Geometry: final body of the model. Coordinates: model frame, mm. A direction names the side the tool comes from. Give positions to 0.01 mm unless a question says otherwise; leave off trailing zeros. Write each loop counter-clockwise with the first axis right and the second up, starting at its lowest first coordinate (ties: lowest second). Pieces come first, ordered by that corner, then holes. Notation, with made-up numbers: M 71,86 L 89,86 A26 ccw 89,123 Z; hole C -36,56 d1. An arc over 180 degrees is marked long. Answer as a JSON object with one key per item and string values.
from build123d import *

# Parameters (mm, degrees)
BASE_EXTRUDE_DEPTH  = 60
CUT_EXTRUDE1_DEPTH  = 50
SKETCH3_R           = 9
BOSS_EXTRUDE1_DEPTH = 15


with BuildPart() as part:
    # Sketch1 → Base-Extrude (new body)
    with BuildSketch(Plane.XY):
        with BuildLine():
            Line((15, 0), (135, 0))
            ThreePointArc((135, 0), (145.606601718, 4.393398282), (150, 15))
            Line((150, 15), (150, 85))
            ThreePointArc((150, 85), (145.606601718, 95.606601718), (135, 100))
            Line((135, 100), (15, 100))
            ThreePointArc((15, 100), (4.393398282, 95.606601718), (0, 85))
            Line((0, 85), (0, 15))
            ThreePointArc((0, 15), (4.393398282, 4.393398282), (15, 0))
        make_face()
    extrude(amount=BASE_EXTRUDE_DEPTH)

    # Sketch2 → Cut-Extrude1 (cut)
    with BuildSketch(Plane.XY.offset(60)):
        with BuildLine():
            Line((40, 80), (40, 20))
            ThreePointArc((40, 20), (42.928932188, 12.928932188), (50, 10))
            Line((50, 10), (130, 10))
            ThreePointArc((130, 10), (137.071067812, 12.928932188), (140, 20))
            Line((140, 20), (140, 80))
            ThreePointArc((140, 80), (137.071067812, 87.071067812), (130, 90))
            Line((130, 90), (50, 90))
            ThreePointArc((50, 90), (42.928932188, 87.071067812), (40, 80))
        make_face()
    extrude(amount=-CUT_EXTRUDE1_DEPTH, mode=Mode.SUBTRACT)

    # Sketch3 → Boss-Extrude1 (add)
    with BuildSketch(Plane.XY.offset(60)):
        with Locations(Location((24, 54.61, 0), (0, 0, 180))):
            Circle(SKETCH3_R)
    extrude(amount=BOSS_EXTRUDE1_DEPTH)


solid = part.part
1) Cut plane A-A on y = 28. Return loops of the section in (x, z), and give its area (3 significant figures).
Geometry check:
{"outline": "M 0,0 L 150,0 L 150,60 L 140,60 L 140,10 L 40,10 L 40,60 L 0,60 Z", "area": "4,000 mm2"}
2) Cut plane B-B on x = 24. Return loops of the section in (y, z).
Geometry check:
{"outline": "M 0,0 L 100,0 L 100,60 L 63.61,60 L 63.61,75 L 45.61,75 L 45.61,60 L 0,60 Z"}
3) Cut plane C-C on z = 24.5. Return loops of the section in (x, y).
Geometry check:
{"outline": "M 0,15 A15 ccw 15,0 L 135,0 A15 ccw 150,15 L 150,85 A15 ccw 135,100 L 15,100 A15 ccw 0,85 Z; hole M 40,20 A10 ccw 50,10 L 130,10 A10 ccw 140,20 L 140,80 A10 ccw 130,90 L 50,90 A10 ccw 40,80 Z"}
4) Set-up query: faces 5 (the flat face through (74, 0, 30)), 6 (the cylindrical face through (136.99, 12.85, 35.35)). Return all of +Z, -Z, +X, -X, +Y, -Y with unobstructed straight access to the full face (end or side cutting, diameter ignored); none if empty.
Geometry check:
{"face 5": "+Z, -Z, +X, -X, -Y", "face 6": "+Z"}
5) Pull-direction query (X, two-part tool) for faces 1 (the cylindrical face through (4.51, 95.72, 29.58)), 2 (the flat face through (24, 54, 75)), 3 (the flat face through (91, 90, 35)), 4 (the cylindrical face through (145.49, 4.28, 29.58)); classes: pulls with the +X half, pulls with the -X half, needs draft (parallel to the pull), parting line crosses it, or undercut.
Geometry check:
{"face 1": "pulls with the -X half", "face 2": "needs draft", "face 3": "undercut", "face 4": "pulls with the +X half"}
6) Line query: line 1 (Y direction, x = 114, z = 50); line 2 (X direction, y = 68, z = 23.5); line 3 (Z direction, x = 29.5, y = 82). Output: solid intervals per line, ascending. Write a range as from..to.
Geometry check:
{"line 1": "y = 0..10, 90..100", "line 2": "x = 0..40, 140..150", "line 3": "z = 0..60"}
7) Contact query for a flat-ended pin moving along its axis: P1, Ø1.5, axis at x = 110, y = 58, coming from the +Z side. Output: stop coordinate, or through.
Geometry check:
{"P1": "stops at z = 10"}
8) Cut plane D-D on y = 54.61. Return loops of the section in (x, z), and give its area (3 significant figures).
Geometry check:
{"outline": "M 0,0 L 150,0 L 150,60 L 140,60 L 140,10 L 40,10 L 40,60 L 33,60 L 33,75 L 15,75 L 15,60 L 0,60 Z", "area": "4,270 mm2"}
